Part model, mm, in its own coordinate system. A direction names the side the tool comes from. Give positions to 0.01 mm unless a question says otherwise; leave off trailing zeros. Write each loop counter-clockwise with the first axis right and the second up, starting at its lowest first coordinate (ties: lowest second). Pieces come first, ordered by that corner, then holes. Notation, with made-up numbers: M 14.25,88 L 48.25,88 A10 cw 48.25,93 Z; hole C 26,6 d1. An arc over 180 degrees is marked long. Write item = value, one per line. Start each with the question number.
from build123d import *

# Parameters (mm, degrees)
SKETCH_1_R      = 2.75
EXTRUDE_1_DEPTH = 10
SKETCH_2_R      = 36.51
EXTRUDE_2_DEPTH = 1.5
SKETCH_3_R      = 6
EXTRUDE_3_DEPTH = 30
EXTRUDE_4_DEPTH = 55


with BuildPart() as part:
    # Эскиз1 → Вытянуть1 (new body)
    with BuildSketch(Plane(origin=(0, 0, 0), x_dir=(1, 0, 0), z_dir=(0, 1, 0))):
        with BuildLine():
            Line((-37, 42.5), (37, 42.5))
            ThreePointArc((37, 42.5), (40.889087297, 40.889087297), (42.5, 37))
            Line((42.5, 37), (42.5, -37))
            ThreePointArc((42.5, -37), (40.889087297, -40.889087297), (37, -42.5))
            Line((37, -42.5), (-37, -42.5))
            ThreePointArc((-37, -42.5), (-40.889087297, -40.889087297), (-42.5, -37))
            Line((-42.5, -37), (-42.5, 37))
            ThreePointArc((-42.5, 37), (-40.889087297, 40.889087297), (-37, 42.5))
        make_face()
        with Locations(Location((-34.8, 34.8, 0), (0, 0, 270))):
            Circle(SKETCH_1_R, mode=Mode.SUBTRACT)
        with Locations(Location((34.8, 34.8, 0), (0, 0, 90))):
            Circle(SKETCH_1_R, mode=Mode.SUBTRACT)
        with Locations(Location((34.8, -34.8, 0), (0, 0, 270))):
            Circle(SKETCH_1_R, mode=Mode.SUBTRACT)
        with Locations(Location((-34.8, -34.8, 0), (0, 0, 90))):
            Circle(SKETCH_1_R, mode=Mode.SUBTRACT)
    extrude(amount=EXTRUDE_1_DEPTH)

    # Эскиз2 → Вытянуть2 (add)
    with BuildSketch(Plane(origin=(0, 10, 0), x_dir=(1, 0, 0), z_dir=(0, 1, 0))):
        with Locations(Location((0, 0, 0), (0, 0, 90))):
            Circle(SKETCH_2_R)
    extrude(amount=EXTRUDE_2_DEPTH)

    # Эскиз3 → Вытянуть3 (add)
    with BuildSketch(Plane(origin=(0, 11.5, 0), x_dir=(1, 0, 0), z_dir=(0, 1, 0))):
        with Locations(Location((0, 0, 0), (0, 0, 270))):
            Circle(SKETCH_3_R)
    extrude(amount=EXTRUDE_3_DEPTH)

    # Эскиз4 → Вытянуть4 (add)
    with BuildSketch(Plane.XZ):
        with BuildLine():
            Line((-42.755134635, 23.986897935), (-42.755134635, -23.986897935))
            ThreePointArc((-42.755134635, -23.986897935), (-42.243466041, -25.322888065), (-40.970265008, -25.975294003))
            ThreePointArc((-40.970265008, -25.975294003), (-31.02184563, -30.739107233), (-26.258032399, -40.687526612))
            ThreePointArc((-26.258032399, -40.687526612), (-25.605626461, -41.960727645), (-24.269636331, -42.472396239))
            Line((-24.269636331, -42.472396239), (23.75936706, -42.472396239))
            ThreePointArc((23.75936706, -42.472396239), (25.09535719, -41.960727645), (25.747763128, -40.687526612))
            ThreePointArc((25.747763128, -40.687526612), (30.585250737, -30.585250737), (40.687526612, -25.747763128))
            ThreePointArc((40.687526612, -25.747763128), (41.960727645, -25.09535719), (42.472396239, -23.75936706))
            Line((42.472396239, -23.75936706), (42.472396239, 23.75936706))
            ThreePointArc((42.472396239, 23.75936706), (41.960727645, 25.09535719), (40.687526612, 25.747763128))
            ThreePointArc((40.687526612, 25.747763128), (30.585250737, 30.585250737), (25.747763128, 40.687526612))
            ThreePointArc((25.747763128, 40.687526612), (25.09535719, 41.960727645), (23.75936706, 42.472396239))
            Line((23.75936706, 42.472396239), (-24.269636331, 42.472396239))
            ThreePointArc((-24.269636331, 42.472396239), (-25.605626461, 41.960727645), (-26.258032399, 40.687526612))
            ThreePointArc((-26.258032399, 40.687526612), (-31.02184563, 30.739107233), (-40.970265008, 25.975294003))
            ThreePointArc((-40.970265008, 25.975294003), (-42.243466041, 25.322888065), (-42.755134635, 23.986897935))
        make_face()
    extrude(amount=EXTRUDE_4_DEPTH)


solid = part.part
Q1. Slice it at A-A (x = -34.8). Give the cut face in (y, z).
Q2. Slice it at C-C (z = -34.8). Give the cut face in (x, y), and give its area (3 significant figures).
Q3. Tool access for faces 1 (the face through (30.7, -27.12, 30.47)), 2 (the face through (-10.967, 10.74, -34.824)), 3 (the face through (30.47, -27.12, -30.7)), 4 (the face through (-31, 0, 31)), 5 (the face through (-31.13, -27.12, -30.63)): list every direction of +Z, -Z, +X, -X, +Y, -Y with a clear straight run to the whole face (end or side of a thin tool).
Q4. Two-plate mould, pull along X, no slides. Class faces 6 (the face through (-40.93, 4.93, -40.85)), 7 (the face through (40.93, 4.93, 40.85)), 8 (the face through (-33.127, 4.93, 36.982)): +X half, -X half, draft (parallel to the pull), parting line (faces both ways), or undercut.
Q5. Drop flat-ended pins along their axis: P1, Ø7, axis at x = 34.8, z = 34.8, coming from the -Y side; P2, Ø1.5, axis at y = -35, z = -29, coming from the -X side; P3, Ø5, axis at y = 3, z = 18, coming from the -X side; P4, Ø4.5, axis at x = 34.8, z = -34.8, coming from the +Y side. Give the stop position or say it passes through.
Q6. Probe line 1 along X through (y, z) = (4.5, 34.8); line 2 along Z through (x, y) = (-34, 4); line 3 along Z through (x, y) = (-24.5, -19.5). List the from-to ranges inside material, lowest first.
Q7. Slice it at B-B (y = -30.5). Give the cut face in (x, z), and give its area (3 significant figures).
Working result:
q1.outline = M -55,-27.91 L 0,-27.91 L 0,-32.05 L 10,-32.05 L 10,-11.04 L 11.5,-11.04 L 11.5,11.04 L 10,11.04 L 10,32.05 L 0,32.05 L 0,27.91 L -55,27.91 Z; M 0,-42.5 L 10,-42.5 L 10,-37.55 L 0,-37.55 Z; M 0,37.55 L 10,37.55 L 10,42.5 L 0,42.5 Z
q2.outline = M -42.5,0 L -37.55,0 L -37.55,10 L -42.5,10 Z; M -32.05,0 L -28.04,0 L -28.04,-55 L 27.51,-55 L 27.51,0 L 32.05,0 L 32.05,10 L 11.04,10 L 11.04,11.5 L -11.04,11.5 L -11.04,10 L -32.05,10 Z; M 37.55,0 L 42.5,0 L 42.5,10 L 37.55,10 Z
q2.area = 3,830 mm2
q3.face_1 = +Z, +X, -Y
q3.face_2 = +Y
q3.face_3 = -Z, +X, -Y
q3.face_4 = -Y
q3.face_5 = -Z, -X, -Y
q4.face_6 = -X half
q4.face_7 = +X half
q4.face_8 = undercut
q5.P1 = 0
q5.P2 = -34.21
q5.P3 = -42.5
q5.P4 = through
q6.line_1 = -42.5 to -37.55, -32.05 to 32.05, 37.55 to 42.5
q6.line_2 = -42.5 to -37.43, -32.17 to 32.17, 37.43 to 42.5
q6.line_3 = -42.46 to 42.46
q7.outline = M -42.76,-23.99 A2 ccw -40.97,-25.98 A16.59 cw -26.26,-40.69 A2 ccw -24.27,-42.47 L 23.76,-42.47 A2 ccw 25.75,-40.69 A16.85 cw 40.69,-25.75 A2 ccw 42.47,-23.76 L 42.47,23.76 A2 ccw 40.69,25.75 A16.85 cw 25.75,40.69 A2 ccw 23.76,42.47 L -24.27,42.47 A2 ccw -26.26,40.69 A16.59 cw -40.97,25.98 A2 ccw -42.76,23.99 Z
q7.area = 6,360 mm2
